```python
from build123d import *

# Parameters (mm, degrees)
F0_W     = 116.554148
F0_H     = 116.554148
F1_DEPTH = 50
F2_R     = 16
F3_DEPTH = 25


with BuildPart() as f1:
    # F0 (on Front) → F1 (new body)
    with BuildSketch(Plane.XZ):
        Rectangle(F0_W, F0_H)
    extrude(amount=F1_DEPTH)

    # F2 (on face) → F3 (cut)
    with BuildSketch(Plane.YZ.offset(58.277074)):
        with Locations((-25, 0)):
            Circle(F2_R)
    extrude(amount=-F3_DEPTH, mode=Mode.SUBTRACT)


solid = f1.part
```
The listing builds one solid part. Answer for the finished solid, in the listing's coordinates (mm). A direction names the side the tool comes from. Coordinates: 2 decimals unless noted, no trailing zeros. Write each loop counter-clockwise with the first axis right and the second up, starting at its lowest first coordinate (ties: lowest second). Pieces come first, ordered by that corner, then holes.
Q1. Section B-B, the plane y = -15 is taken. Write down the section's boundary in (x, z).
Returned:
outline: (-58.28, -58.28) - (58.28, -58.28) - (58.28, -12.49) - (33.28, -12.49) - (33.28, 12.49) - (58.28, 12.49) - (58.28, 58.28) - (-58.28, 58.28) - close
Q2. The mould has two halves that part along Z. Classify faces 1 (the flat face through (-1, -25, 58.277)), 2 (the flat face through (-58.277, -25, -1)), 3 (the flat face through (33.277, -25, 0)): released by +Z, released by -Z, zero draft, split by the parting line, or undercut.
Returned:
face 1: released by +Z
face 2: zero draft
face 3: undercut
Q3. Section A-A, the plane x = 40 is taken. Write down the section's boundary in (y, z).
Returned:
outline: (-50, -58.28) - (0, -58.28) - (0, 58.28) - (-50, 58.28) - close; hole circle Ø32 at (-25, 0)
Q4. Find the intervals of material crossed by line 1 along Z through (x, y) = (39, -25); line 2 along X through (y, z) = (-21, -13); line 3 along Z through (x, y) = (35.5, -38.5), in increasing order.
Returned:
line 1: z = -58.28 to -16, 16 to 58.28
line 2: x = -58.28 to 33.28
line 3: z = -58.28 to -8.59, 8.59 to 58.28
Q5. Which of the six approach directions +Z, -Z, +X, -X, +Y, -Y give full straight-line access (tool end or side, diameter ignored) to faces 4 (the flat face through (58.277, -41.3, -0.8)), 5 (the cylindrical face through (45.95, -28.47, -15.62))?
Returned:
face 4: +Z, -Z, +X, +Y, -Y
face 5: +X
Q6. Section C-C, the plane z = 0 is taken. Write down the section's boundary in (x, y).
Returned:
outline: (-58.28, -50) - (58.28, -50) - (58.28, -41) - (33.28, -41) - (33.28, -9) - (58.28, -9) - (58.28, 0) - (-58.28, 0) - close
Q7. Given P1, Ø19, axis at y = -25, z = 0, coming from the +X side, flat-ended and moving along its own axis, determine where the tip first touches the part or whether it passes through.
Returned:
P1: stops at x = 33.28
